The model under review builds one solid part; all positions refer to its coordinate system, in mm. A direction names the side the tool comes from. Give positions to 0.01 mm unless a question says otherwise; leave off trailing zeros. Loops run counter-clockwise (first coordinate to the right, second up) from the corner with the lowest first, then second, coordinate; pieces in that order, holes last. Notation, with made-up numbers: M 38.5,57 L 97.5,57 A27 ccw 97.5,76 Z; hole C 23,76.5 d8. An arc over 180 degrees is marked long. Put each result on its own line as item: value. Start each with the question number.
```python
from build123d import *

# Parameters (mm, degrees)
CONG_1_R = 1


with BuildPart() as part:
    # Esquisse1 → Révolution1 (revolve)
    with BuildSketch(Plane.XY, mode=Mode.PRIVATE) as r_volution1_sk:
        with BuildLine():
            Line((-4.5, 39.289558898), (-4.5, 37.789558898))
            Line((-4.5, 37.789558898), (-6, 37.789558898))
            Line((-6, 37.789558898), (-6, 36.289558898))
            Line((-6, 36.289558898), (-4, 36.289558898))
            Line((-4, 36.289558898), (-4, 31.289558898))
            Line((-4, 31.289558898), (-4.5, 31.289558898))
            Line((-4.5, 31.289558898), (-4.5, 29.789558898))
            Line((-4.5, 29.789558898), (0, 29.789558898))
            Line((0, 29.789558898), (0, 48.289558898))
            Line((0, 48.289558898), (-4.5, 48.289558898))
            Line((-4.5, 48.289558898), (-4.5, 47.226812831))
            ThreePointArc((-4.5, 47.226812831), (-6, 43.258185864), (-4.5, 39.289558898))
        make_face()
    revolve(r_volution1_sk.sketch.rotate(Axis((0, 0, 0), (0, 1, 0)), 270), axis=Axis((0, 0, 0), (0, 1, 0)))

    # Congé1
    cong_1_edges = [part.edges().sort_by_distance(p)[0] for p in [
        (0, 29.789558898, 4.5),
    ]]
    fillet(cong_1_edges, radius=CONG_1_R)


solid = part.part
```
Item 1: Draft analysis for pull direction Y (two halves, no side actions). For faces 1 (the flat face through (0, 29.79, 0)), 2 (the cylindrical face through (-1.802, 37.029, -5.723)), 3 (the flat face through (3, 31.29, -3)), state which applies: +Y half, -Y half, draft (parallel to the pull), parting line (faces both ways), or undercut.
Item 2: Clearance check with flat-ended pins moving along their axes: pin 1 Ø2 at (x, y) = (3.5, 33.5) entering from -Z; pin 2 Ø6 at (x, y) = (-4.5, 41.5) entering from +Z; pin 3 Ø6 at (x, y) = (-3.5, 36) entering from +Z. State where each tip first meets the part, or that it passes through.
Item 3: To check wall thickness, follow L1, parallel to Y at x = 4.75, z = 2.5; L2, parallel to Y at x = 4.5, z = -3.5; L3, parallel to X at y = 46, z = 4.75. State the ranges of each line that lie inside material, in increasing order. Write a range as [from, to].
Item 4: Consider section B-B, the plane x = 0. Write out the cut boundary in (y, z).
Item 5: Consider section A-A, the plane z = 0. Write out the cut boundary in (x, y).
Item 6: Consider section C-C, the plane y = 43.25. Write out the cut boundary in (x, z), plus the area to 3 significant figures.
Item 7: Tool access review of faces 4 (the flat face through (3.92, 36.29, 1.42)), 5 (the cylindrical face through (-1.352, 47.751, -4.292)), 6 (the cylindrical face through (-1.352, 31.036, -4.292)), 7 (the flat face through (0, 48.29, 0)): name each direction out of +Z, -Z, +X, -X, +Y, -Y from which nothing blocks a thin tool from reaching the whole face with its end or side.
Item 8: Consider section D-D, the plane z = 4.75. Write out the cut boundary in (x, y), plus the area to 3 significant figures.
Report:
1. face 1: -Y half
1. face 2: draft
1. face 3: undercut
2. pin 1: z = -3.12
2. pin 2: z = 5.71
2. pin 3: z = 5.98
3. L1: [36.29, 37.79], [40.58, 45.94]
3. L2: [36.29, 37.79], [41.39, 45.13]
3. L3: [-2.43, 2.43]
4. outline: M 29.79,-3.5 A1 ccw 30.79,-4.5 L 31.29,-4.5 L 31.29,-4 L 36.29,-4 L 36.29,-6 L 37.79,-6 L 37.79,-4.5 L 39.29,-4.5 A6 ccw 47.23,-4.5 L 48.29,-4.5 L 48.29,4.5 L 47.23,4.5 A6 ccw 39.29,4.5 L 37.79,4.5 L 37.79,6 L 36.29,6 L 36.29,4 L 31.29,4 L 31.29,4.5 L 30.79,4.5 A1 ccw 29.79,3.5 Z
5. outline: M -6,36.29 L -4,36.29 L -4,31.29 L -4.5,31.29 L -4.5,30.79 A1 ccw -3.5,29.79 L 3.5,29.79 A1 ccw 4.5,30.79 L 4.5,31.29 L 4,31.29 L 4,36.29 L 6,36.29 L 6,37.79 L 4.5,37.79 L 4.5,39.29 A6 ccw 4.5,47.23 L 4.5,48.29 L -4.5,48.29 L -4.5,47.23 A6 ccw -4.5,39.29 L -4.5,37.79 L -6,37.79 Z
6. outline: C 0,0 d12
6. area: 113 mm²
7. face 4: none
7. face 5: +Y
7. face 6: -Y
7. face 7: +Z, -Z, +X, -X, +Y
8. outline: M -3.67,36.29 L 3.67,36.29 L 3.67,37.79 L -3.67,37.79 Z; C 0,43.26 d7.33
8. area: 53.2 mm²
